Can you work these out from the drawing? Everything is in mm from the part's minimum corner. A direction names the side the tool comes from. Give positions to 0.01 mm unless a question says otherwise; leave off trailing zeros. Order: outer loops, then holes, each group sorted by start corner. A loop starts at its lowest first (then second) coordinate and runs counter-clockwise, first axis right, second up. Notation, with made-up numbers: M 80,-28 L 98,-28 A14 ccw 98,-24 Z; hole C -2,51.25 d6. An arc over 180 degrees is marked long. Answer as a JSON object with one key per item and string values.
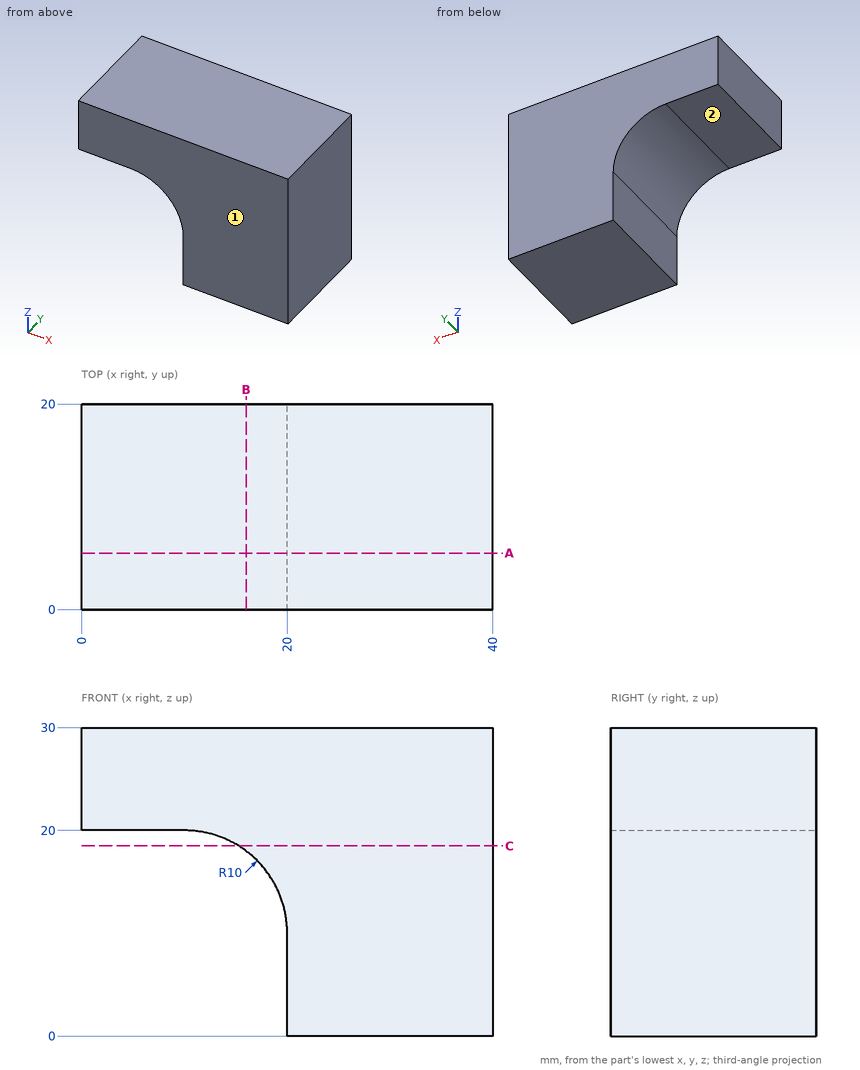
1) I want a section at B-B on x = 16. Write out the boundary of the cut face in (y, z), and give its area (3 significant figures).
Results found:
{"outline": "M 0,18 L 20,18 L 20,30 L 0,30 Z", "area": "240 mm²"}
2) I'm going to push flat-ended pins straight in: pin 1 Ø3 at (x, y) = (3.5, 12.5) entering from -Z; pin 2 Ø12 at (y, z) = (8.5, 21) entering from -X; pin 3 Ø6 at (y, z) = (15, 5) entering from -X. Where does each tip first touch, or does it pass through?
Results found:
{"pin 1": "stops at z = 20", "pin 2": "stops at x = 0", "pin 3": "stops at x = 20"}
3) I need wall thicknesses on L1, parallel to X at y = 9, z = 1.75; L2, parallel to Z at x = 2, y = 4; L3, parallel to Z at x = 14, y = 15. Which ranges of each line are inside material? Lowest first, please.
Results found:
{"L1": "x = 20 to 40", "L2": "z = 20 to 30", "L3": "z = 19.17 to 30"}
4) I want a section at A-A on y = 5.5. Write out the boundary of the cut face in (x, z), and give its area (3 significant figures).
Results found:
{"outline": "M 0,20 L 10,20 A10 cw 20,10 L 20,0 L 40,0 L 40,30 L 0,30 Z", "area": "821 mm²"}
5) I want a section at C-C on z = 18.5. Write out the boundary of the cut face in (x, y).
Results found:
{"outline": "M 15.27,0 L 40,0 L 40,20 L 15.27,20 Z"}
6) For the marked faces 1 and 2, which set-ups out of +Z, -Z, +X, -X, +Y, -Y let a thin tool reach every point of the face, with its end or its side?
Results found:
{"face 1": "+Z, -Z, +X, -X, -Y", "face 2": "-Z, -X, +Y, -Y"}
